The model under review builds one solid part; all positions refer to its coordinate system, in mm. A direction names the side the tool comes from. Round coordinates to 2 decimals unless told otherwise and drop trailing zeros. Write each loop counter-clockwise with the first axis right and the second up, starting at its lowest first coordinate (ties: lowest second). Pieces come first, ordered by that corner, then holes. Notation, with made-up numbers: (21.5, 76.25) - (31.5, 76.25) arc R22 ccw to (31.5, 114.25) - close; hole circle Ø7 at (53, 16.25). An arc over 180 degrees is marked (long way). Return JSON: item names as keys, results as strings.
from build123d import *

# Parameters (mm, degrees)
F0_W     = 18.5
F0_H     = 10
F0_W_2   = 13.5
F0_H_2   = 7
F1_DEPTH = 9
F3_DEPTH = 3
F2_W     = 25
F2_H     = 1
F2_H_2   = 5
F2_R     = 1.75
F4_DEPTH = 1
F5_R     = 2.75
F6_DEPTH = 1
F7_W     = 2
F7_H     = 1.75
F8_DEPTH = 0.25


with BuildPart() as f1:
    # F0 (on Top) → F1 (new body)
    with BuildSketch(Plane.XY):
        Rectangle(F0_W, F0_H)
        Rectangle(F0_W_2, F0_H_2, mode=Mode.SUBTRACT)
    extrude(amount=F1_DEPTH)

    # F2 (on face) → F3 (join)
    with BuildSketch(Plane(origin=(0, 0, 0), x_dir=(1, 0, 0), z_dir=(0, 0, -1))):
        Polygon((9.25, -5), (13.75, -5), (13.75, 1.4), (13, 2), (9.25, 5), align=None)
    extrude(amount=-F3_DEPTH)

    # F2 (on face) → F4 (join)
    with BuildSketch(Plane(origin=(0, 0, 0), x_dir=(1, 0, 0), z_dir=(0, 0, -1))):
        Polygon((13.75, -5), (14.25, -5), (14.25, -4), (14.25, 1), (13.75, 1.4), align=None)
        Polygon((39.25, -4), (39.25, -5), (40.25, -5), (40.25, 2), (13, 2), (13.75, 1.4), (14.25, 1), (39.25, 1), align=None)
        with Locations((26.75, -4.5)):
            Rectangle(F2_W, F2_H)
        with Locations((26.75, -1.5)):
            Rectangle(F2_W, F2_H_2)
        with Locations((16.75, -1.5)):
            Circle(F2_R, mode=Mode.SUBTRACT)
        with Locations((36.75, -1.5)):
            Circle(F2_R, mode=Mode.SUBTRACT)
    extrude(amount=-F4_DEPTH)

    # F5 (on face) → F6 (join)
    with BuildSketch(Plane(origin=(0, 5, 0), x_dir=(-1, 0, 0), z_dir=(0, 1, 0))):
        Polygon((-13.75, 1), (-14.25, 1), (-39.25, 1), (-40.25, 1), (-40.25, 0), (9.25, 0), (9.25, 9), (-9.25, 9), (-9.25, 3), (-9.25, 1), align=None)
        with BuildLine():
            Line((-39.25, 1), (-14.25, 1))
            Line((-14.25, 1), (-14.25, 9))
            Line((-14.25, 9), (-23.5096296508, 9))
            ThreePointArc((-23.5096296508, 9), (-23.502408305, 8.8750926958), (-23.5, 8.75))
            ThreePointArc((-23.5, 8.75), (-26.8750926958, 5.502408305), (-29.9903703492, 9))
            Line((-29.9903703492, 9), (-35.25, 9))
            ThreePointArc((-35.25, 9), (-36.3135467206, 4.7809953781), (-39.25, 1.5703297516))
            Line((-39.25, 1.5703297516), (-39.25, 1))
        make_face()
        with Locations((-31.525, 3.975)):
            Circle(F5_R, mode=Mode.SUBTRACT)
        with Locations((-22.025, 3.975)):
            Circle(F5_R, mode=Mode.SUBTRACT)
        Polygon((-14.25, 9), (-14.25, 1), (-13.75, 1), (-13.75, 3), (-9.25, 3), (-9.25, 9), align=None)
        with BuildLine():
            Line((-40.25, 1), (-39.25, 1))
            Line((-39.25, 1), (-39.25, 1.5703297516))
            ThreePointArc((-39.25, 1.5703297516), (-39.7407688872, 1.2689793045), (-40.25, 1))
        make_face()
    extrude(amount=-F6_DEPTH)

    # F7 (on face) → F8 (join)
    with BuildSketch(Plane.XY.offset(9)):
        with Locations((0, -4.125)):
            Rectangle(F7_W, F7_H)
    extrude(amount=F8_DEPTH)


solid = f1.part
(1) Add section C-C (z = 0.5). Write out the cut boundary in (x, y), plus the area to 3 significant figures.
Filled in:
{"outline": "(-9.25, -5) - (9.25, -5) - (13, -2) - (40.25, -2) - (40.25, 5) - (-9.25, 5) - close; hole (-6.75, -3.5) - (6.75, -3.5) - (6.75, 3.5) - (-6.75, 3.5) - close; hole circle Ø3.5 at (16.75, 1.5); hole circle Ø3.5 at (36.75, 1.5)", "area": "294 mm2"}
(2) Mouldability with a two-part tool opening along X and no side actions: class faces 4 (the cylindrical face through (34.272, 4.507, 4.096)), 5 (the cylindrical face through (19.4, 4.5, 4.8)), 6 (the flat face through (13.75, 1, 2)), 7 (the flat face through (10, 5, 4)) as released by +X, released by -X, zero draft, split by the parting line, or undercut.
Filled in:
{"face 4": "undercut", "face 5": "undercut", "face 6": "released by +X", "face 7": "zero draft"}
(3) Add section B-B (y = 1.5). Write out the cut boundary in (x, z), plus the area to 3 significant figures.
Filled in:
{"outline": "(-9.25, 0) - (-6.75, 0) - (-6.75, 9) - (-9.25, 9) - close; (6.75, 0) - (15, 0) - (15, 1) - (13.75, 1) - (13.75, 3) - (9.25, 3) - (9.25, 9) - (6.75, 9) - close; (18.5, 0) - (35, 0) - (35, 1) - (18.5, 1) - close; (38.5, 0) - (40.25, 0) - (40.25, 1) - (38.5, 1) - close", "area": "78.0 mm2"}
(4) Wall thickness on line 1 (X direction, y = 1.5, z = 0.5); line 2 (X direction, y = -0.5, z = 7.75); line 3 (Y direction, x = 16.75, z = 0.65): over which ranges is each line inside the solid? List them lowest first.
Filled in:
{"line 1": "x = -9.25 to -6.75, 6.75 to 15, 18.5 to 35, 38.5 to 40.25", "line 2": "x = -9.25 to -6.75, 6.75 to 9.25", "line 3": "y = -2 to -0.25, 3.25 to 5"}
(5) Add section A-A (x = 16.75). Write out the cut boundary in (y, z).
Filled in:
{"outline": "(-2, 0) - (-0.25, 0) - (-0.25, 1) - (-2, 1) - close; (3.25, 0) - (5, 0) - (5, 9) - (4, 9) - (4, 1) - (3.25, 1) - close"}
(6) For faces 1 (the flat face through (11, 0, 3)), 2 (the flat face through (26.8, -2, 0.5)), 3 (the flat face through (0, 3.5, 4)), list the 3-axis set-ups (+Z, -Z, +X, -X, +Y, -Y) from which the entire face can be reached by the end or side of a thin tool; tool diameter is ignored.
Filled in:
{"face 1": "+Z, +X, -Y", "face 2": "+Z, -Z, +X, -Y", "face 3": "+Z, -Z"}
(7) Clearance check with flat-ended pins moving along their axes: pin 1 Ø1.6 at (y, z) = (0.5, 2.5) entering from +X; pin 2 Ø1 at (x, z) = (15.5, 3.5) entering from -Y; pin 3 Ø5 at (y, z) = (3, 5.5) entering from +X. State where each tip first meets the part, or that it passes through.
Filled in:
{"pin 1": "stops at x = 13.75", "pin 2": "stops at y = 4", "pin 3": "stops at x = 37.39"}
(8) Add section D-D (x = 26.75). Write out the cut boundary in (y, z).
Filled in:
{"outline": "(-2, 0) - (5, 0) - (5, 5.5) - (4, 5.5) - (4, 1) - (-2, 1) - close"}
